Check sheet for the modelled part. Datum: model origin and axes. Units: mm. Face numbers are marked on the shaded views. A direction names the side the tool comes from. Give positions to 0.01 mm unless a question says otherwise; leave off trailing zeros. Loops run counter-clockwise (first coordinate to the right, second up) from the corner with the lowest first, then second, coordinate; pieces in that order, holes last. Notation, with made-up numbers: M -20.75,-34.75 L 29.25,-34.75 A6 ccw 29.25,-29.75 Z; hole C -19,53 d4. An arc over 180 degrees is marked long. Write each question's results on one line, items separated by ' | '. Start each with the question number.
1. Sectioned sample at C-C on y = -44. Record the cut outline in (x, z), and give its area (3 significant figures).
2. Sectioned sample at B-B on z = 37. Record the cut outline in (x, y).
3. Material ranges on line 1 along Y through (x, z) = (-29.5, -7.5); line 2 along Z through (x, y) = (-3.5, -28); line 3 along Z through (x, y) = (-16, -8.5), recorded low to high.
4. Sectioned sample at A-A on x = -30.5. Record the cut outline in (y, z), and give its area (3 significant figures).
5. Sectioned sample at D-D on x = -36. Record the cut outline in (y, z).
6. Draft check along Z on the marked faces 5, 6, 7 and 8. Enter one of: pulls with the +Z half, pulls with the -Z half, needs draft (parallel to the pull), parting line crosses it, or undercut.
7. Go/stop test with flat-tipped pins: pin 1 (4 mm diameter, centred on x = -45.5, y = -38, fed in from -Z); pin 2 (7.5 mm diameter, centred on x = -24.5, z = -13, fed in from -Y); pin 3 (12.5 mm diameter, centred on y = -20, z = -10.5, fed in from +X). Record where each tip stops, or that it passes through.
8. Tool access check on the marked faces 1, 2, 3 and 4. Record the directions out of +Z, -Z, +X, -X, +Y, -Y that give a thin tool (end or side, any length) a straight path to the whole face; none if there is none.
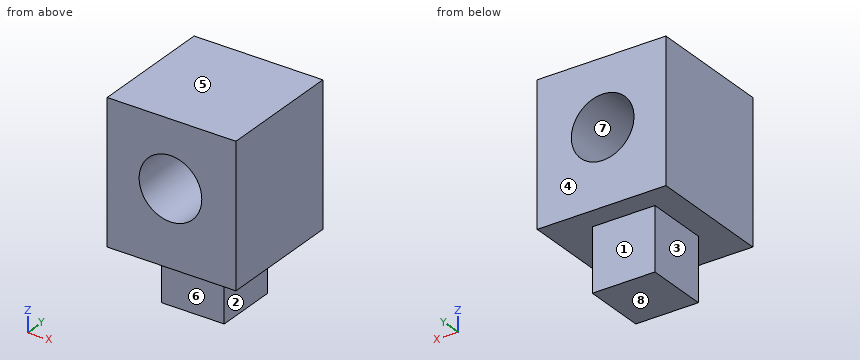
```python
from build123d import *

# Parameters (mm, degrees)
F0_W     = 52.19904
F0_H     = 57.19075
F1_DEPTH = 50.8
F3_D     = 25.4
F4_W     = 25.4
F4_H     = 25.4
F5_DEPTH = 25.4


with BuildPart() as f1:
    # F0 (on Front) → F1 (new body)
    with BuildSketch(Plane.XZ):
        with Locations((-26.09952, 28.595375)):
            Rectangle(F0_W, F0_H)
    extrude(amount=F1_DEPTH)

    # F3 (through all)
    with Locations(Plane(origin=(0, 0, 0), x_dir=(-1, 0, 0), z_dir=(0, 1, 0))):
        with Locations((26.545139, 30.546911)):
            Hole(F3_D / 2)

    # F4 (on face) → F5 (join)
    with BuildSketch(Plane(origin=(0, 0, 0), x_dir=(1, 0, 0), z_dir=(0, 0, -1))):
        with Locations((-28.771738, 21.757494)):
            Rectangle(F4_W, F4_H)
    extrude(amount=F5_DEPTH)


solid = f1.part
```
Output values:
1) outline: M -52.2,0 L 0,0 L 0,57.19 L -52.2,57.19 Z; hole C -26.55,30.55 d25.4 | area: 2,480 mm2
2) outline: M -52.2,-50.8 L -37.48,-50.8 L -37.48,0 L -52.2,0 Z; M -15.61,-50.8 L 0,-50.8 L 0,0 L -15.61,0 Z
3) line 1: -34.46 to -9.06 | line 2: 0 to 57.19 | line 3: 0 to 23.47, 37.62 to 57.19
4) outline: M -50.8,0 L -34.46,0 L -34.46,-25.4 L -9.06,-25.4 L -9.06,0 L 0,0 L 0,18.48 L -50.8,18.48 Z; M -50.8,42.62 L 0,42.62 L 0,57.19 L -50.8,57.19 Z | area: 2,320 mm2
5) outline: M -50.8,0 L -34.46,0 L -34.46,-25.4 L -9.06,-25.4 L -9.06,0 L 0,0 L 0,22.07 L -50.8,22.07 Z; M -50.8,39.03 L 0,39.03 L 0,57.19 L -50.8,57.19 Z
6) face 5: pulls with the +Z half | face 6: needs draft | face 7: undercut | face 8: pulls with the -Z half
7) pin 1: z = 0 | pin 2: y = -34.46 | pin 3: x = -16.07
8) face 1: -Z, +X, -X, +Y | face 2: -Z, +X, +Y, -Y | face 3: -Z, -X, +Y, -Y | face 4: +Z, -Z, +X, -X, +Y
